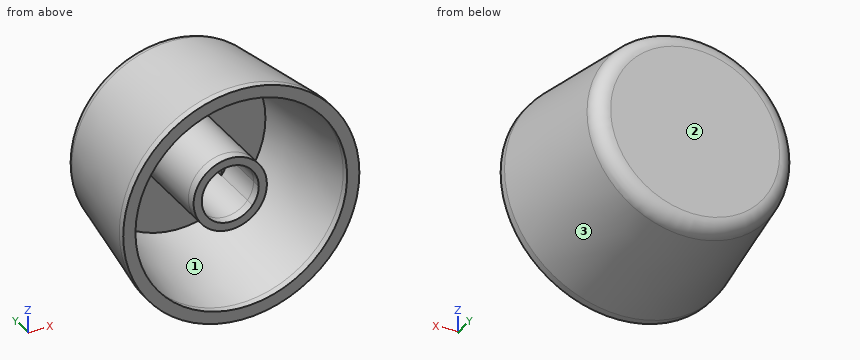
from build123d import *
from build123d import SkipClean  # not in build123d's __all__

# Parameters (mm, degrees)
F2_R     = 2
F4_DEPTH = 6
F5_DEPTH = 10
F6_DEPTH = 0.9
F3_R     = 4.4988269867
F7_DEPTH = 1.2


with BuildPart() as f1:
    # F0 (on Top) → F1 (revolve)
    with BuildSketch(Plane.XY):
        Polygon((0.6408938694, 2.8410089679), (0.6408938694, 16.7043862722), (-11.46528483, 16.7043862722), (-13.8516243371, 0), (-12.3516243371, 0), (-10.3318675491, 14.1383057447), (-3.8579331173, 14.1383057447), (-3.8579331173, 2.8410089679), align=None)
    revolve(axis=Axis((0.6408938694, 3.1900271702, 0), (0, -1, 0)))

    # F2
    f2_edges = [f1.edges().sort_by_distance(p)[0] for p in [
        (12.747073, 16.704386, 0),
    ]]
    fillet(f2_edges, radius=F2_R)

    # F3 (on face) → F4 (cut)
    with BuildSketch(Plane.XZ.offset(-2.8410089679)):
        with BuildLine():
            ThreePointArc((3.3910251828, -2.1648967087), (3.9481177503, -1.1455436271), (4.1408938694, 0))
            ThreePointArc((4.1408938694, 0), (3.9481177503, 1.1455436271), (3.3910251828, 2.1648967087))
            Line((3.3910251828, 2.1648967087), (3.3910251828, -2.1648967087))
        make_face()
        with BuildLine():
            Line((3.3910251828, -2.1648967087), (3.3910251828, 2.1648967087))
            ThreePointArc((3.3910251828, 2.1648967087), (-2.8591061306, 0), (3.3910251828, -2.1648967087))
        make_face()
    extrude(amount=-F4_DEPTH, mode=Mode.SUBTRACT)

    # F3 (on face) → F5 (cut)
    with BuildSketch(Plane.XZ.offset(-2.8410089679)):
        with BuildLine():
            Line((3.3910251828, -2.1648967087), (3.3910251828, 2.1648967087))
            ThreePointArc((3.3910251828, 2.1648967087), (-2.8591061306, 0), (3.3910251828, -2.1648967087))
        make_face()
    extrude(amount=-F5_DEPTH, mode=Mode.SUBTRACT)

    # F6 (add): a face of the model
    f6_faces = [f1.faces().sort_by_distance(p)[0] for p in [
        (14.72350176, 0, 0),
    ]]
    extrude(f6_faces, amount=F6_DEPTH)

    # F3 (on face) → F7 (join)
    with BuildSketch(Plane.XZ.offset(-2.8410089679)):
        with Locations((0.6408938694, 0)):
            Circle(F3_R)
        with BuildLine():
            ThreePointArc((3.3910251828, 2.1648967087), (3.9481177503, 1.1455436271), (4.1408938694, 0))
            ThreePointArc((4.1408938694, 0), (3.9481177503, -1.1455436271), (3.3910251828, -2.1648967087))
            ThreePointArc((3.3910251828, -2.1648967087), (-2.8591061306, 0), (3.3910251828, 2.1648967087))
        make_face(mode=Mode.SUBTRACT)
    with SkipClean():  # cleaning this boolean's faces spoils the solid; the shape is the same uncleaned
        extrude(amount=F7_DEPTH)


solid = f1.part
Input: part model. Units: mm. Frame: model coordinates. Face numbers are marked on the shaded views. Give positions to 0.01 mm unless a question says otherwise; leave off trailing zeros. Answer as a JSON object with one key per item and string values. Group by question number.
Item 1: Pin query (flat end, axial travel): P1, Ø4, axis at y = 2.5, z = 0, coming from the +X side; P2, Ø8, axis at x = 3.5, y = 3, coming from the -Z side; P3, Ø3, axis at x = 5.5, y = 8, coming from the +Z side; P4, Ø3, axis at x = 0, z = 1, coming from the -Y side. Return the tip coordinate at first contact, or that it passes through.
Item 2: Line query: probe 1 along X at (y, z) = (-0.6, 0); probe 2 along X at (y, z) = (2.3, 0); probe 3 along Z at (x, y) = (4.75, 8). Output: solid intervals per line, ascending.
Item 3: Pull-direction query (X, two-part tool) for the marked faces 1, 2 and 3; classes: released by +X, released by -X, zero draft, split by the parting line, or undercut.
Checks:
{
 "1": {"P1": "stops at x = 15.06", "P2": "stops at z = -14.49", "P3": "stops at z = 12.98", "P4": "stops at y = 12.84"},
 "2": {"probe 1": "x = -13.85 to -12.35, 13.63 to 15.13", "probe 2": "x = -13.52 to -12.02, -3.86 to -2.86, 4.14 to 5.14, 13.3 to 14.8", "probe 3": "z = -12.7 to -11.11, -1.83 to 1.83, 11.11 to 12.7"},
 "3": {"face 1": "undercut", "face 2": "zero draft", "face 3": "split by the parting line"}
}
